Here's how the part is built. I have some questions about the finished solid (model axes, mm). A direction names the side the tool comes from. Round coordinates to 2 decimals unless told otherwise and drop trailing zeros. Loops run counter-clockwise (first coordinate to the right, second up) from the corner with the lowest first, then second, coordinate; pieces in that order, holes last. Notation, with made-up numbers: M 62,70.25 L 92,70.25 A10 ccw 92,89.25 Z; hole C 64,-38.5 d5. An arc over 180 degrees is marked long. Write each question's results on one line, items separated by ' | '. Start each with the question number.
```python
from build123d import *

# Parameters (mm, degrees)
BOSS_EXTRU_1_DEPTH      = 15
CONG_1_R                = 3
ENL_V_MAT_EXTRU_1_DEPTH = 0.5


with BuildPart() as part:
    # Esquisse1 → Boss.-Extru.1 (new body)
    with BuildSketch(Plane(origin=(0, 0, 0), x_dir=(1, 0, 0), z_dir=(0, 1, 0))):
        with BuildLine():
            Line((-12, -22), (12, -22))
            ThreePointArc((12, -22), (19.071067812, -19.071067812), (22, -12))
            Line((22, -12), (22, 12))
            ThreePointArc((22, 12), (19.071067812, 19.071067812), (12, 22))
            Line((12, 22), (-12, 22))
            ThreePointArc((-12, 22), (-19.071067812, 19.071067812), (-22, 12))
            Line((-22, 12), (-22, -12))
            ThreePointArc((-22, -12), (-19.071067812, -19.071067812), (-12, -22))
        make_face()
    extrude(amount=BOSS_EXTRU_1_DEPTH)

    # Congé1
    cong_1_edges = [part.edges().sort_by_distance(p)[0] for p in [
        (19.071067812, 15, 19.071067812),
        (22, 15, 0),
        (19.071067812, 15, -19.071067812),
        (0, 15, -22),
        (-19.071067812, 15, -19.071067812),
        (-22, 15, 0),
        (-19.071067812, 15, 19.071067812),
        (0, 15, 22),
    ]]
    fillet(cong_1_edges, radius=CONG_1_R)

    # Esquisse2 → Enlèv. mat.-Extru.1 (cut)
    with BuildSketch(Plane(origin=(0, 15, 0), x_dir=(1, 0, 0), z_dir=(0, 1, 0))):
        with BuildLine():
            Line((-12, 7.018114977), (-12, -7.018114977))
            ThreePointArc((-12, -7.018114977), (-11.726888823, -7.46367245), (-11.205914151, -7.422483019))
            Line((-11.205914151, -7.422483019), (-2.112012116, -0.808736084))
            ThreePointArc((-2.112012116, -0.808736084), (-1.700183814, 0), (-2.112012116, 0.808736084))
            Line((-2.112012116, 0.808736084), (-11.205914151, 7.422483019))
            ThreePointArc((-11.205914151, 7.422483019), (-11.726888823, 7.46367245), (-12, 7.018114977))
        make_face()
        with BuildLine():
            Line((1, 6), (11, 6))
            ThreePointArc((11, 6), (11.707106781, 5.707106781), (12, 5))
            Line((12, 5), (12, -5))
            ThreePointArc((12, -5), (11.707106781, -5.707106781), (11, -6))
            Line((11, -6), (1, -6))
            ThreePointArc((1, -6), (0.292893219, -5.707106781), (0, -5))
            Line((0, -5), (0, 5))
            ThreePointArc((0, 5), (0.292893219, 5.707106781), (1, 6))
        make_face()
    extrude(amount=-ENL_V_MAT_EXTRU_1_DEPTH, mode=Mode.SUBTRACT)


solid = part.part
```
1. I want a section at C-C on z = -3. List the corners of the cut face in (x, y) for me (3 decimals), plus the area to 3 significant figures.
2. I want a section at B-B on z = 3.5. List the corners of the cut face in (x, y) for me, plus the area to 3 significant figures.
3. I need wall thicknesses on line 1 along Y through (x, z) = (-10, -3.5); line 2 along Z through (x, y) = (12.5, 10.5). Which ranges of each line are inside material? Lowest first, please.
4. If we mould it in two halves opening along Z, with no side actions, what happens to faces 3 (the face through (18.99, 5.92, 19.15)), 4 (the face through (-8, 14.5, 0)), 5 (the face through (22, 6, 0))? For each: released by +Z, released by -Z, zero draft, split by the parting line, or undercut.
5. I want a section at A-A on y = 4.25. List the corners of the cut face in (x, z) for me.
6. For pin 1 (3 mm diameter, centred on x = 17.5, y = 9, fed in from -Z); pin 2 (0.6 mm diameter, centred on y = 15, z = -3, fed in from +X); pin 3 (1 mm diameter, centred on y = 2, z = -15, fed in from -X), each with a flat end and sliding along its axis, tell me the tip position at first contact or that it passes through.
7. Which directions (+Z, -Z, +X, -X, +Y, -Y) give clear straight access to the entire face, cutting with the end or side of a thin tool? Please do faces 1 (the face through (6, 14.5, 0)), 2 (the face through (-0.3, 15, -0.3)).
Outcome:
1) outline: M -22,0 L 22,0 L 22,12 A3 ccw 19,15 L 12,15 L 12,14.5 L 0,14.5 L 0,15 L -5.125,15 L -5.125,14.5 L -12,14.5 L -12,15 L -19,15 A3 ccw -22,12 Z | area: 647 mm2
2) outline: M -22,0 L 22,0 L 22,12 A3 ccw 19,15 L 12,15 L 12,14.5 L 0,14.5 L 0,15 L -5.81,15 L -5.81,14.5 L -12,14.5 L -12,15 L -19,15 A3 ccw -22,12 Z | area: 647 mm2
3) line 1: 0 to 14.5 | line 2: -21.99 to 21.99
4) face 3: released by +Z | face 4: undercut | face 5: zero draft
5) outline: M -22,-12 A10 ccw -12,-22 L 12,-22 A10 ccw 22,-12 L 22,12 A10 ccw 12,22 L -12,22 A10 ccw -22,12 Z
6) pin 1: z = -21.17 | pin 2: x = 20.31 | pin 3: x = -21.68
7) face 1: +Y | face 2: +Z, -Z, +X, -X, +Y
